Answer from the drawing. Dimensions are ordinates in mm from the lowest x, y and z of the part. Round coordinates to 2 decimals unless told otherwise and drop trailing zeros. Write each loop counter-clockwise with the first axis right and the second up, starting at its lowest first coordinate (ties: lowest second). Pieces come first, ordered by that corner, then holes. Notation, with made-up numbers: (47, 66) -> (106, 66) arc R16 cw to (106, 85) -> close; hole circle Ø2 at (-29, -37). An arc over 180 degrees is marked (long way). Return JSON: item names as keys, results as strings. Group by question number.
(1) Straight lines are drawn through the part: line 1 (X direction, y = 78.5, z = 36.5); line 2 (Z direction, x = 3, y = 665); line 3 (Z direction, x = 11.5, y = 383). For each, find the intervals that lie inside material, in ascending order.
(2) A cutting plane is placed at A-A on z = 100. Give the vertices of the cut face in (x, y), then the cut area to 3 significant figures.
(3) A cutting plane is placed at B-B on y = 375. Give the vertices of the cut face in (x, z).
(4) Given pin 1 (3 mm diameter, centred on x = 27, z = 75, fed in from -Y); pin 2 (12 mm diameter, centred on y = 158.5, z = 41.5, fed in from -X), each flat-ended and moving along its own axis, determine where each tip first touches the part or whether it passes through.
(5) A cutting plane is placed at C-C on z = 22.5. Give the vertices of the cut face in (x, y), then the cut area to 3 significant figures.
(6) The mould has two halves that part along Y. Classify the marked faces 1 and 2: released by +Y, released by -Y, zero draft, split by the parting line, or undercut.
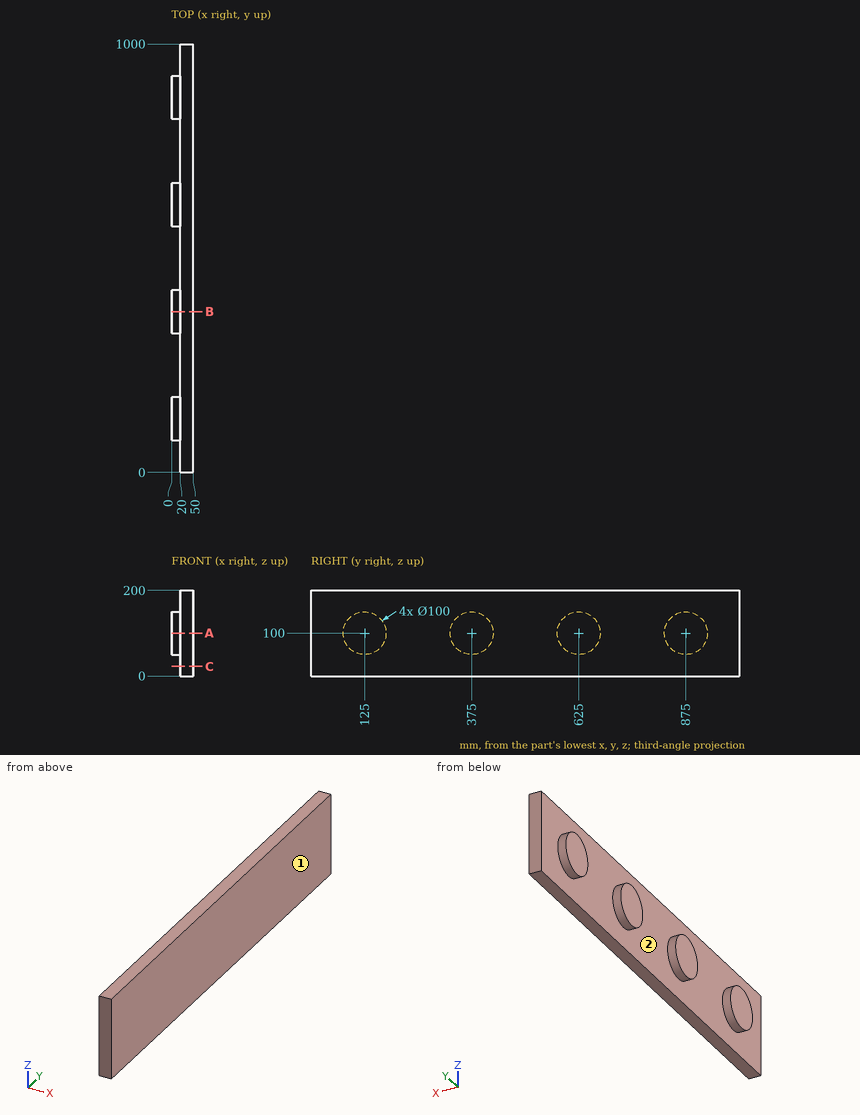
Checks:
{
 "1": {"line 1": "x = 20 to 50", "line 2": "z = 70 to 130", "line 3": "z = 50.64 to 149.36"},
 "2": {"outline": "(0, 75) -> (20, 75) -> (20, 0) -> (50, 0) -> (50, 1000) -> (20, 1000) -> (20, 925) -> (0, 925) -> (0, 825) -> (20, 825) -> (20, 675) -> (0, 675) -> (0, 575) -> (20, 575) -> (20, 425) -> (0, 425) -> (0, 325) -> (20, 325) -> (20, 175) -> (0, 175) -> close", "area": "38,000 mm^2"},
 "3": {"outline": "(0, 50) -> (20, 50) -> (20, 0) -> (50, 0) -> (50, 200) -> (20, 200) -> (20, 150) -> (0, 150) -> close"},
 "4": {"pin 1": "stops at y = 0", "pin 2": "stops at x = 20"},
 "5": {"outline": "(20, 0) -> (50, 0) -> (50, 1000) -> (20, 1000) -> close", "area": "30,000 mm^2"},
 "6": {"face 1": "zero draft", "face 2": "undercut"}
}
